The listing builds one solid part. Answer for the finished solid, in the listing's coordinates (mm). A direction names the side the tool comes from. Give positions to 0.01 mm unless a question says otherwise; leave off trailing zeros. Loops run counter-clockwise (first coordinate to the right, second up) from the corner with the lowest first, then second, coordinate; pieces in that order, holes last. Notation, with made-up numbers: (82.5, 39.5) - (109.5, 39.5) arc R27 ccw to (109.5, 77.5) - close; hole circle Ø6 at (14.25, 75.5). An arc over 180 degrees is marked (long way). Write each question's results on one line, items separated by ' | '.
Autodesk Inventor part; units mm, degrees
ref_plane "YZ Plane" through (0, 0, 0) normal (1, 0, 0) x (0, 1, 0)
ref_plane "XZ Plane" through (0, 0, 0) normal (0, 1, 0) x (-1, 0, 0)
ref_plane "XY Plane" through (0, 0, 0) normal (0, 0, 1) x (1, 0, 0)
sketch "Sketch1" plane through (0, 0, 0) normal (0, 0, 1) x (1, 0, 0)
  line L0 (-28.575, -28.575) -> (28.575, -28.575)
  line L1 (28.575, -28.575) -> (28.575, 28.575)
  line L2 (28.575, 28.575) -> (-28.575, 28.575)
  line L3 (-28.575, 28.575) -> (-28.575, -28.575)
  line L4 (-28.575, -28.575) -> (28.575, 28.575) construction
  line L5 (28.575, -28.575) -> (-28.575, 28.575) construction
  point P0 (0, 0)
  dimension "d0" = 57.15
  dimension "d1" = 57.15
extrude "Extrusion1" add sketch "Sketch1" along normal blind 12.7
sketch "Sketch2" plane through (0, 0, 12.7) normal (0, 0, 1) x (1, 0, 0)
  line L0 (-21.15, -21.15) -> (21.15, -21.15)
  line L1 (21.15, -21.15) -> (21.15, 21.15)
  line L2 (21.15, 21.15) -> (-21.15, 21.15)
  line L3 (-21.15, 21.15) -> (-21.15, -21.15)
  line L4 (-21.15, -21.15) -> (21.15, 21.15) construction
  line L5 (21.15, -21.15) -> (-21.15, 21.15) construction
  point P0 (0, 0)
  dimension "d4" = 42.3
  dimension "d5" = 42.3
extrude "Extrusion2" cut sketch "Sketch2" against normal blind 6.35
sketch "Sketch3" plane through (-21.15, 21.15, 12.7) normal (0, -1, 0) x (1, 0, 0)
  line L0 (0, 0) -> (42.3, 0)
  line L1 (0, 0) -> (0, -6.35)
  line L2 (0, -6.35) -> (42.3, -6.35)
  line L3 (42.3, 0) -> (42.3, -6.35)
  line L4 (21.15, -6.35) -> (24.325, -6.35)
  line L5 (24.325, -6.35) -> (24.325, 0)
  line L6 (24.325, 0) -> (21.15, 0)
  line L7 (21.15, -6.35) -> (17.975, -6.35)
  line L8 (17.975, -6.35) -> (17.975, 0)
  line L9 (17.975, 0) -> (21.15, 0)
  point P0 (21.15, -12.7)
  dimension "d10" = 17.975
  dimension "d11" = 17.975
extrude "Extrusion3" cut sketch "Sketch3" against normal up to next contours L0 L5 L2 L8
sketch "Sketch4" plane through (0, 0, 12.7) normal (0, 0, 1) x (1, 0, 0)
  line L0 (28.575, -28.575) -> (28.575, 28.575)
  line L1 (28.575, 28.575) -> (3.175, 28.575)
  line L2 (28.575, 28.575) -> (-28.575, -28.575) construction
  line L3 (-28.575, 28.575) -> (28.575, -28.575) construction
  line L4 (28.575, 24.8625) -> (24.8625, 24.8625) construction
  line L5 (-24.8625, -24.8625) -> (24.8625, -24.8625) construction
  line L6 (24.8625, -24.8625) -> (24.8625, 24.8625) construction
  line L7 (24.8625, 24.8625) -> (-24.8625, 24.8625) construction
  line L8 (-24.8625, 24.8625) -> (-24.8625, -24.8625) construction
  line L9 (-24.8625, -24.8625) -> (24.8625, 24.8625) construction
  line L10 (24.8625, -24.8625) -> (-24.8625, 24.8625) construction
  point P0 (0, 0)
  dimension "d14" = 3.7125
hole "Hole1" at (-24.8625, 24.8625, 12.7) at (24.8625, 24.8625, 12.7) at (24.8625, -24.8625, 12.7) at (-24.8625, -24.8625, 12.7) direction (0, 0, -1) diameter 4.4958 end through all
sketch "Sketch5" plane through (-28.575, -28.575, 0) normal (0, -1, 0) x (1, 0, 0)
  line L0 (57.15, 0) -> (57.15, 12.7)
  line L1 (0, 12.7) -> (57.15, 12.7)
  line L2 (0, 0) -> (0, 12.7)
  line L3 (3.9568, 4.7625) -> (48.9174, 4.7625) construction
  point P0 (28.575, 0)
  point P1 (10.16, 4.7625)
  point P2 (46.99, 4.7625)
  dimension "d22" = 7.9375
  dimension "d23" = 10.16
  dimension "d24" = 10.16
hole "Hole2" at (-18.415, -28.575, 4.7625) at (18.415, -28.575, 4.7625) direction (0, 1, 0) diameter 4.3434 depth 6.35 tip angle 118
equation "\"d1\" = d0"
equation "\"d11\" = d10"
properties part number "NEMA_17-back" material "Aluminum 6061"
Item 1: For faces 5 (the face through (20.535, -25.356, 5.233)), 6 (the face through (-3.175, 25, 9)), 7 (the face through (21.15, 0, 10)), determine the directions among +Z, -Z, +X, -X, +Y, -Y from which every point of the face is accessible in a straight line to the end or side of a thin tool.
Values found:
face 5: -Y | face 6: +Z, +Y | face 7: +Z
Item 2: Find the intervals of material crossed by line 1 along Y through (x, z) = (-6.5, 10.5) (3 decimals); line 2 along X through (y, z) = (23, 9) (3 decimals); line 3 along Y through (x, z) = (23.5, 7) (3 decimals), in increasing order. Write a range as [from, to].
Values found:
line 1: y = [-28.575, -21.15], [21.15, 28.575] | line 2: x = [-28.575, -26.121], [-23.604, -3.175], [3.175, 23.604], [26.121, 28.575] | line 3: y = [-28.575, -26.65], [-23.075, 23.075], [26.65, 28.575]
Item 3: A cutting plane is placed at D-D, the plane x = 1.5. Determine the outline of the cut face in (y, z) (3 decimals), plus the area to 3 significant figures.
Values found:
outline: (-28.575, 0) - (28.575, 0) - (28.575, 6.35) - (-21.15, 6.35) - (-21.15, 12.7) - (-28.575, 12.7) - close | area: 410 mm²
Item 4: Flat-ended cylindrical pins translate along their axes: P1, Ø1.9, axis at x = -1.5, z = 10.5, coming from the +Y side; P2, Ø4, axis at x = 18.42, z = 4.76, coming from the -Y side; P3, Ø12.5, axis at x = -9.5, y = 2, coming from the +Z side. Find the tip coordinate at first contact, or state that the pin passes through.
Values found:
P1: stops at y = -21.15 | P2: stops at y = -22.13 | P3: stops at z = 6.35
Item 5: For a pull along Y with two mould halves and no side action, classify faces 1 (the face through (28.575, 0, 6)), 2 (the face through (-25.538, -27.007, 6.261)), 3 (the face through (0, -28.575, 6)), 4 (the face through (0, 28.575, 6)) as released by +Y, released by -Y, zero draft, split by the parting line, or undercut.
Values found:
face 1: zero draft | face 2: undercut | face 3: released by -Y | face 4: released by +Y
Item 6: A cutting plane is placed at A-A, the plane y = 16. Determine the outline of the cut face in (x, z) (3 decimals).
Values found:
outline: (-28.575, 0) - (28.575, 0) - (28.575, 12.7) - (21.15, 12.7) - (21.15, 6.35) - (-21.15, 6.35) - (-21.15, 12.7) - (-28.575, 12.7) - close
Item 7: A cutting plane is placed at C-C, the plane z = 1.5. Determine the outline of the cut face in (x, y) (1 decimal).
Values found:
outline: (-28.6, -28.6) - (28.6, -28.6) - (28.6, 28.6) - (-28.6, 28.6) - close; hole circle Ø4.5 at (-24.9, -24.9); hole circle Ø4.5 at (-24.9, 24.9); hole circle Ø4.5 at (24.9, -24.9); hole circle Ø4.5 at (24.9, 24.9)
